Work out the finished part from the listing and answer in its coordinate system (mm). Face numbers are marked on the shaded views. A direction names the side the tool comes from. Round coordinates to 2 decimals unless told otherwise and drop trailing zeros. Loops run counter-clockwise (first coordinate to the right, second up) from the corner with the lowest first, then second, coordinate; pieces in that order, holes last.
```python
from build123d import *

# Parameters (mm, degrees)
SKETCH2_W           = 127
SKETCH2_H           = 76.2
SKETCH2_R           = 6.35
BOSS_EXTRUDE1_DEPTH = 38.1
SKETCH3_W           = 38.1
SKETCH3_H           = 76.2
CUT_EXTRUDE1_DEPTH  = 25.4
FILLET1_R           = 12.7
CHAMFER1_SIZE       = 3.175


with BuildPart() as part:
    # Sketch2 → Boss-Extrude1 (new body)
    with BuildSketch(Plane(origin=(0, 0, 0), x_dir=(1, 0, 0), z_dir=(0, 1, 0))):
        Rectangle(SKETCH2_W, SKETCH2_H)
        with Locations((-44.45, 19.05)):
            Circle(SKETCH2_R, mode=Mode.SUBTRACT)
        with Locations((44.45, 19.05)):
            Circle(SKETCH2_R, mode=Mode.SUBTRACT)
        with Locations((44.45, -19.05)):
            Circle(SKETCH2_R, mode=Mode.SUBTRACT)
        with Locations((-44.45, -19.05)):
            Circle(SKETCH2_R, mode=Mode.SUBTRACT)
    extrude(amount=BOSS_EXTRUDE1_DEPTH)

    # Sketch3 → Cut-Extrude1 (cut)
    with BuildSketch(Plane(origin=(0, 38.1, 0), x_dir=(1, 0, 0), z_dir=(0, 1, 0))):
        Rectangle(SKETCH3_W, SKETCH3_H)
    extrude(amount=-CUT_EXTRUDE1_DEPTH, mode=Mode.SUBTRACT)

    # Fillet1
    fillet1_edges = [part.edges().sort_by_distance(p)[0] for p in [
        (63.5, 19.05, 38.1),
        (-63.5, 19.05, 38.1),
        (-63.5, 19.05, -38.1),
        (63.5, 19.05, -38.1),
    ]]
    fillet(fillet1_edges, radius=FILLET1_R)

    # Chamfer1
    chamfer1_edges = [part.edges().sort_by_distance(p)[0] for p in [
        (34.925, 38.1, 38.1),
        (-34.925, 38.1, -38.1),
        (19.05, 12.7, 0),
        (19.05, 25.4, -38.1),
        (0, 12.7, 38.1),
        (19.05, 25.4, 38.1),
        (-19.05, 12.7, 0),
        (-19.05, 25.4, 38.1),
        (0, 12.7, -38.1),
        (-19.05, 25.4, -38.1),
        (19.05, 38.1, 0),
        (-19.05, 38.1, 0),
        (-34.925, 38.1, 38.1),
        (-63.5, 38.1, 0),
        (-59.780256121, 38.1, -34.380256121),
        (-59.780256121, 38.1, 34.380256121),
        (34.925, 38.1, -38.1),
        (63.5, 38.1, 0),
        (59.780256121, 38.1, 34.380256121),
        (59.780256121, 38.1, -34.380256121),
    ]]
    chamfer(chamfer1_edges, length=CHAMFER1_SIZE)


solid = part.part
```
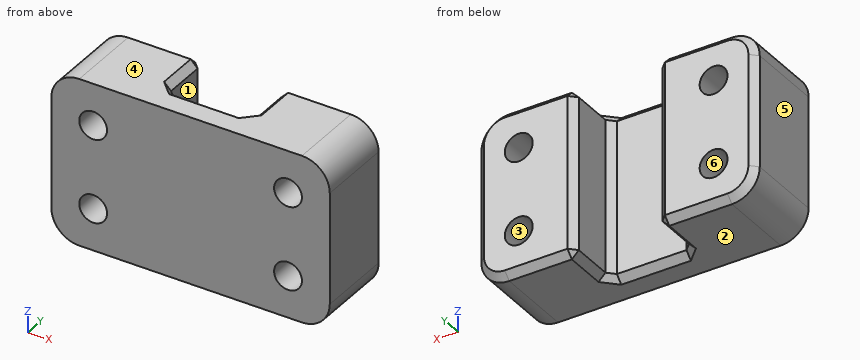
1. Which of the six approach directions +Z, -Z, +X, -X, +Y, -Y give full straight-line access (tool end or side, diameter ignored) to the marked faces 1 and 2?
Answer key:
face 1: +Z, -Z, +Y
face 2: -Z, +X, -X, +Y, -Y
2. Find section B-B (z = -19.05). Write down the section's boundary in (x, y) (3 decimals), then the cut area to 3 significant figures.
Answer key:
outline: (-63.5, 0) - (-50.8, 0) - (-50.8, 38.1) - (-60.325, 38.1) - (-63.5, 34.925) - close; (-38.1, 0) - (38.1, 0) - (38.1, 38.1) - (22.225, 38.1) - (19.05, 34.925) - (19.05, 15.875) - (15.875, 12.7) - (-15.875, 12.7) - (-19.05, 15.875) - (-19.05, 34.925) - (-22.225, 38.1) - (-38.1, 38.1) - close; (50.8, 0) - (63.5, 0) - (63.5, 34.925) - (60.325, 38.1) - (50.8, 38.1) - close
area: 2,890 mm2
3. Find section D-D (z = 1.5). Write down the section's boundary in (x, y) (3 decimals).
Answer key:
outline: (-63.5, 0) - (63.5, 0) - (63.5, 34.925) - (60.325, 38.1) - (22.225, 38.1) - (19.05, 34.925) - (19.05, 15.875) - (15.875, 12.7) - (-15.875, 12.7) - (-19.05, 15.875) - (-19.05, 34.925) - (-22.225, 38.1) - (-60.325, 38.1) - (-63.5, 34.925) - close
4. Find section C-C (x = 44.45). Write down the section's boundary in (y, z) (3 decimals), then the cut area to 3 significant figures.
Answer key:
outline: (0, -38.1) - (34.925, -38.1) - (38.1, -34.925) - (38.1, -25.4) - (0, -25.4) - close; (0, -12.7) - (38.1, -12.7) - (38.1, 12.7) - (0, 12.7) - close; (0, 25.4) - (38.1, 25.4) - (38.1, 34.925) - (34.925, 38.1) - (0, 38.1) - close
area: 1,930 mm2
5. Consider probe 1 along Z at (x, y) = (44.45, 19.5); probe 2 along X at (y, z) = (27, -19); probe 3 along X at (y, z) = (11.5, 19.05). Determine where each line is inside the solid, lowest interval first.
Answer key:
probe 1: z = -38.1 to -25.4, -12.7 to 12.7, 25.4 to 38.1
probe 2: x = -63.5 to -50.8, -38.1 to -19.05, 19.05 to 38.1, 50.8 to 63.5
probe 3: x = -63.5 to -50.8, -38.1 to 38.1, 50.8 to 63.5
6. Given pin 1 (8 mm diameter, centred on x = 6.5, y = 12, fed in from -Z); pin 2 (9.5 mm diameter, centred on x = 3.5, z = 0, fed in from +Y); pin 3 (7.5 mm diameter, centred on x = 44.45, z = -19.05, fed in from -Y), each flat-ended and moving along its own axis, determine where each tip first touches the part or whether it passes through.
Answer key:
pin 1: stops at z = -38.1
pin 2: stops at y = 12.7
pin 3: passes through
7. Determine the mould class of the marked faces 3, 4, 5 and 6 for opening direction Z: +Z half, -Z half, draft (parallel to the pull), parting line (faces both ways), or undercut.
Answer key:
face 3: undercut
face 4: +Z half
face 5: draft
face 6: undercut
8. Find section A-A (y = 25). Write down the section's boundary in (x, z) (3 decimals).
Answer key:
outline: (-63.5, -25.4) arc R12.7 ccw to (-50.8, -38.1) - (-22.225, -38.1) - (-19.05, -34.925) - (-19.05, 34.925) - (-22.225, 38.1) - (-50.8, 38.1) arc R12.7 ccw to (-63.5, 25.4) - close; (19.05, -34.925) - (22.225, -38.1) - (50.8, -38.1) arc R12.7 ccw to (63.5, -25.4) - (63.5, 25.4) arc R12.7 ccw to (50.8, 38.1) - (22.225, 38.1) - (19.05, 34.925) - close; hole circle Ø12.7 at (-44.45, -19.05); hole circle Ø12.7 at (-44.45, 19.05); hole circle Ø12.7 at (44.45, -19.05); hole circle Ø12.7 at (44.45, 19.05)
